Part model, mm, in its own coordinate system. Face numbers are marked on the shaded views. A direction names the side the tool comes from. Give positions to 0.01 mm unless a question says otherwise; leave off trailing zeros. Order: outer loops, then holes, each group sorted by start corner. A loop starts at its lowest first (then second) coordinate and runs counter-clockwise, first axis right, second up. Notation, with made-up numbers: (41.25, -3) - (80.25, -3) arc R24 cw to (80.25, 9) - close; hole circle Ø3 at (-9.75, 5.25). An arc over 180 degrees is marked (long way). Use one line per item in the form item = value. Start each with the question number.
1. Band-saw the part on C-C, the plane z = -10.25. List the corners of the cut face in (x, y) (1 decimal).
2. Pull direction X, two halves, no side cores. Call the marked faces 1, 2 and 3: +X half, -X half, draft (parallel to the pull), parting line (faces both ways), or undercut.
3. Drill centre lines: line 1 (X direction, y = 5, z = -11.5); line 2 (Y direction, x = -3.5, z = 2.5). Where is each one in solid material? Low to high.
4. Pin check, flat tips, straight feed: P1, Ø12.5, axis at x = 4.5, z = 1.5, coming from the +Y side; P2, Ø12, axis at x = -10.5, y = 10, coming from the -Z side. Stop position of each tip, or through.
5. Band-saw the part on D-D, the plane x = 7. List the corners of the cut face in (y, z), plus the area to 3 significant figures.
6. Band-saw the part on A-A, the plane y = 12.5. List the corners of the cut face in (x, z).
7. Tool access for the marked faces 4, 5 and 6: list every direction of +Z, -Z, +X, -X, +Y, -Y with a clear straight run to the whole face (end or side of a thin tool).
from build123d import *

# Parameters (mm, degrees)
BASE_EXTRUDE_DEPTH = 12.7


with BuildPart() as part:
    # Sketch1 → Base-Extrude (new, symmetric)
    with BuildSketch(Plane.XY):
        with BuildLine():
            Line((-11.3109375, 20.6375), (-18.8515625, 20.6375))
            ThreePointArc((-18.8515625, 20.6375), (-20.114411017, 20.114411017), (-20.6375, 18.8515625))
            Line((-20.6375, 18.8515625), (-20.6375, -18.8515625))
            ThreePointArc((-20.6375, -18.8515625), (-20.114411017, -20.114411017), (-18.8515625, -20.6375))
            Line((-18.8515625, -20.6375), (18.8515625, -20.6375))
            ThreePointArc((18.8515625, -20.6375), (20.114411017, -20.114411017), (20.6375, -18.8515625))
            Line((20.6375, -18.8515625), (20.6375, 18.8515625))
            ThreePointArc((20.6375, 18.8515625), (20.114411017, 20.114411017), (18.8515625, 20.6375))
            Line((18.8515625, 20.6375), (11.3109375, 20.6375))
            ThreePointArc((11.3109375, 20.6375), (10.048088983, 20.114411017), (9.525, 18.8515625))
            Line((9.525, 18.8515625), (9.525, 13.49375))
            Line((9.525, 13.49375), (13.096875, 13.49375))
            Line((13.096875, 13.49375), (13.096875, 17.065625))
            Line((13.096875, 17.065625), (17.065625, 17.065625))
            Line((17.065625, 17.065625), (17.065625, -17.065625))
            Line((17.065625, -17.065625), (-17.065625, -17.065625))
            Line((-17.065625, -17.065625), (-17.065625, 17.065625))
            Line((-17.065625, 17.065625), (-13.096875, 17.065625))
            Line((-13.096875, 17.065625), (-13.096875, 13.49375))
            Line((-13.096875, 13.49375), (-9.525, 13.49375))
            Line((-9.525, 13.49375), (-9.525, 18.8515625))
            ThreePointArc((-9.525, 18.8515625), (-10.048088983, 20.114411017), (-11.3109375, 20.6375))
        make_face()
    extrude(amount=BASE_EXTRUDE_DEPTH, both=True)


solid = part.part
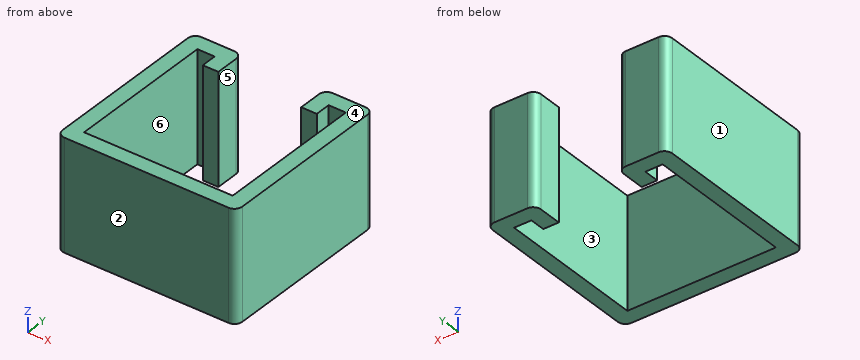
From the geometry:
q1.outline = (-20.6, -18.9) arc R1.8 ccw to (-18.9, -20.6) - (18.9, -20.6) arc R1.8 ccw to (20.6, -18.9) - (20.6, 18.9) arc R1.8 ccw to (18.9, 20.6) - (11.3, 20.6) arc R1.8 ccw to (9.5, 18.9) - (9.5, 13.5) - (13.1, 13.5) - (13.1, 17.1) - (17.1, 17.1) - (17.1, -17.1) - (-17.1, -17.1) - (-17.1, 17.1) - (-13.1, 17.1) - (-13.1, 13.5) - (-9.5, 13.5) - (-9.5, 18.9) arc R1.8 ccw to (-11.3, 20.6) - (-18.9, 20.6) arc R1.8 ccw to (-20.6, 18.9) - close
q2.face_1 = -X half
q2.face_2 = draft
q2.face_3 = undercut
q3.line_1 = -20.64 to -17.07, 17.07 to 20.64
q3.line_2 = -20.64 to -17.07
q4.P1 = 20.55
q4.P2 = -12.7
q5.outline = (-20.64, -12.7) - (-17.07, -12.7) - (-17.07, 12.7) - (-20.64, 12.7) - close
q5.area = 90.7 mm²
q6.outline = (-20.64, -12.7) - (-17.07, -12.7) - (-17.07, 12.7) - (-20.64, 12.7) - close; (17.07, -12.7) - (20.64, -12.7) - (20.64, 12.7) - (17.07, 12.7) - close
q7.face_4 = +Z, +X, -X, +Y, -Y
q7.face_5 = +Z, -Z, +Y
q7.face_6 = +Z, -Z
